Model file for the job. Use its own axes, mm. A direction names the side the tool comes from. Coordinates: 2 decimals unless noted, no trailing zeros. Write each loop counter-clockwise with the first axis right and the second up, starting at its lowest first coordinate (ties: lowest second). Pieces come first, ordered by that corner, then holes. Notation, with made-up numbers: (11, -15) - (25, -15) arc R19 cw to (25, -4) - close; hole circle Ø6 at (-6, 32). An arc over 180 degrees is marked (long way). Put each result on its own line as item: value. Start each with the question number.
1. Drop flat-ended pins along their axis: P1, Ø12, axis at x = 31, y = 47.5, coming from the +Z side; P2, Ø4, axis at x = 29.5, z = 14.5, coming from the +Y side; P3, Ø4.5, axis at x = 17.5, z = 23, coming from the -Y side; P4, Ø13, axis at y = 24.5, z = 20, coming from the -X side. Give the stop position or say it passes through.
2. Pull direction Z, two halves, no side cores. Call faces 1 (the face through (15.029, 2.535, 21.425)), 2 (the face through (50, 53, 21)), 3 (the face through (56, 38, 37)), 4 (the face through (60, 27, 18)): released by +Z, released by -Z, zero draft, split by the parting line, or undercut.
3. Saw through at A-A, the plane x = 47.5. Write the cut outline in (y, z), plus the area to 3 significant figures.
4. Saw through at B-B, the plane y = 45.5. Write the cut outline in (x, z), plus the area to 4 significant figures.
5. Drill centre lines: L1, parallel to X at y = 14, z = 30; L2, parallel to X at y = 1, z = 23; L3, parallel to X at y = 13, z = 31. Where is each one in solid material? Low to high. Write a range as from..to.
6. Saw through at C-C, the plane z = 27. Write the cut outline in (x, y), plus the area to 3 significant figures.
7. Which spindle directions (+Z, -Z, +X, -X, +Y, -Y) get a long thin tool onto all of the face, cutting with end or side? Do faces 5 (the face through (50, 50, 29)), 6 (the face through (10, 28, 17)), 7 (the face through (24, 40, 14)). Say none if no direction does.
8. Saw through at D-D, the plane y = 33. Write the cut outline in (x, z).
Autodesk Inventor part; units mm, degrees
ref_plane "YZ Plane" through (0, 0, 0) normal (1, 0, 0) x (0, 1, 0)
ref_plane "XZ Plane" through (0, 0, 0) normal (0, 1, 0) x (-1, 0, 0)
ref_plane "XY Plane" through (0, 0, 0) normal (0, 0, 1) x (1, 0, 0)
sketch "Sketch3" plane through (0, 0, 0) normal (0, 0, 1) x (1, 0, 0)
  line L0 (0, 0) -> (0, 55)
  line L1 (0, 55) -> (17.5, 55)
  line L2 (17.5, 55) -> (17.5, 40)
  line L3 (17.5, 40) -> (45, 40)
  line L4 (45, 40) -> (45, 55)
  line L5 (10.4377, 0) -> (0, 0)
  line L6 (45, 55) -> (60, 55)
  line L7 (60, 55) -> (60, 0)
  line L8 (60, 0) -> (0, 0)
  dimension "d7" = 55
  dimension "d8" = 17.5
  dimension "d12" = 15
  dimension "d13" = 27.5
  dimension "d14" = 15
  dimension "d15" = 55
  dimension "d16" = 60
extrude "Extrusion2" add sketch "Sketch3" along normal blind 5
sketch "Sketch4" plane through (0, 55, 0) normal (0, 1, 0) x (1, 0, 0)
  line L0 (17.5, -5) -> (0, -5)
  line L1 (0, -37) -> (17.5, -37)
  line L2 (17.5, -37) -> (17.5, -5)
  line L3 (17.5, -5) -> (0, -5)
  line L4 (0, -5) -> (0, -37)
  point P0 (0, 0)
  dimension "d20" = 32
  dimension "d21" = 17.5
extrude "Extrusion3" add sketch "Sketch4" against normal blind 55
sketch "Sketch5" plane through (45, 55, 0) normal (0, 1, 0) x (1, 0, 0)
  line L0 (15, 0) -> (15, -5)
  line L1 (-0.039, -37) -> (15, -37)
  line L2 (15, -37) -> (15, -5)
  line L3 (15, -5) -> (-0.039, -5)
  line L4 (-0.039, -5) -> (-0.039, -37)
  point P0 (-45, 0)
  dimension "d24" = 32
extrude "Extrusion4" add sketch "Sketch5" against normal blind 5
sketch "Sketch7" plane through (17.5, 40, 0) normal (0, 1, 0) x (1, 0, 0)
  line L0 (0, -5) -> (0, -37)
  line L1 (27.5, -5) -> (0, -5)
  line L2 (0, -37) -> (7.5, -37)
  line L3 (7.5, -37) -> (7.5, -5)
  line L4 (7.5, -5) -> (0, -5)
  line L5 (0, -5) -> (0, -37)
  point P0 (-17.5, 0)
  dimension "d27" = 7.5
extrude "Extrusion5" add sketch "Sketch7" against normal blind 40
sketch "Sketch8" plane through (0, 0, 5) normal (0, 0, 1) x (1, 0, 0)
  line L0 (25, 0) -> (60, 0)
  line L1 (60, 0) -> (60, 50)
  line L2 (25, 0) -> (60, 0)
  line L3 (60, 0) -> (60, 5)
  line L4 (60, 5) -> (25, 5)
  line L5 (25, 5) -> (25, 0)
  point P0 (0, 0)
  dimension "d30" = 5
extrude "Extrusion6" add sketch "Sketch8" along normal blind 32
sketch "Sketch9" plane through (0, 0, 5) normal (0, 0, 1) x (1, 0, 0)
  line L0 (60, 50) -> (45, 50)
  line L1 (60, 50) -> (55, 50)
  line L2 (55, 50) -> (55, 0)
  line L3 (55, 0) -> (60, 0)
  line L4 (60, 0) -> (60, 50)
  point P0 (0, 0)
  dimension "d31" = 32
  dimension "d33" = 50
  dimension "d34" = 5
extrude "Extrusion7" add sketch "Sketch9" along normal blind 32
sketch "Sketch10" plane through (0, 55, 0) normal (0, 1, 0) x (1, 0, 0)
  line L0 (10, -30.5) -> (5, -30.5)
  line L1 (5, -30.5) -> (5, -4.5)
  line L2 (5, -4.5) -> (10, -4.5)
  line L3 (10, -4.5) -> (10, -30.5)
  line L4 (17.5, 0) -> (17.5, -37)
  line L5 (0, 0) -> (17.5, 0)
  line L6 (0, 0) -> (0, -37)
  dimension "d45" = 5
  dimension "d46" = 26
  dimension "d47" = 7.5
  dimension "d48" = 4.5
extrude "Extrusion8" cut sketch "Sketch10" against normal blind 60
sketch "Sketch11" plane through (0, 55, 0) normal (0, 1, 0) x (1, 0, 0)
  line L0 (5, -4.5) -> (5, -30.5)
  line L1 (0, 0) -> (0, -37)
  line L2 (5, -28) -> (0, -28)
  line L3 (0, -28) -> (0, -7)
  line L4 (0, -7) -> (5, -7)
  line L5 (5, -7) -> (5, -28)
  line L6 (0, -37) -> (17.5, -37)
  point P0 (5, -35)
  dimension "d52" = 21
  dimension "d53" = 9
extrude "Extrusion9" cut sketch "Sketch11" against normal blind 60
sketch "Sketch12" plane through (0, 0, 0) normal (0, -1, 0) x (1, 0, 0)
  circle A0 centre (17.5, 10.5) radius 2.5
  circle A1 centre (17.5, 23) radius 2.5
  line L0 (10, 30.5) -> (10, 4.5)
  line L1 (0, 37) -> (60, 37)
  line L2 (60, 0) -> (0, 0)
  point P0 (10, 35)
  point P1 (25, 35)
  dimension "d56" = 5
  dimension "d57" = 5
  dimension "d58" = 7.5
  dimension "d59" = 7.5
  dimension "d78" = 14
  dimension "d79" = 12.5
hole "Hole1" at (17.5, 0, 10.5) at (17.5, 0, 23) direction (0, 1, 0) diameter 5.86 depth 5 tip angle 118
sketch "Sketch14" plane through (0, 55, 37) normal (0, 0, 1) x (1, 0, 0)
  line L0 (55, -5) -> (55, -50)
  line L1 (60, 0) -> (60, -55)
  line L2 (55, -50) -> (60, -50)
  line L3 (60, -50) -> (60, -45)
  line L4 (60, -45) -> (55, -45)
  line L5 (55, -45) -> (55, -50)
  point P0 (0, -55)
  dimension "d69" = 5
extrude "Extrusion10" cut sketch "Sketch14" along normal mid plane 64
sketch "Sketch20" plane through (45, 55, 0) normal (0, 1, 0) x (1, 0, 0)
  line L0 (-0.039, -37) -> (-0.039, -5)
  line L1 (0, 0) -> (15, 0)
  line L2 (-0.039, -21) -> (10, -21)
  line L3 (10, -21) -> (10, 0)
  line L4 (10, 0) -> (-0.039, 0)
  line L5 (-0.039, 0) -> (-0.039, -21)
  line L6 (15, 0) -> (15, -37)
  point P0 (-45, 0)
  dimension "d77" = 5
extrude "Extrusion12" cut sketch "Sketch20" against normal blind 15
properties part number "Holder" material "Iron, Cast"
Final values:
1. P1: passes through
1. P2: stops at y = 5
1. P3: stops at y = 5.41
1. P4: stops at x = 10
2. face 1: undercut
2. face 2: released by -Z
2. face 3: released by +Z
2. face 4: zero draft
3. outline: (0, 0) - (40, 0) - (40, 5) - (5, 5) - (5, 37) - (0, 37) - close; (50, 21) - (55, 21) - (55, 37) - (50, 37) - close
3. area: 440 mm²
4. outline: (0, 0) - (17.5, 0) - (17.5, 37) - (0, 37) - (0, 28) - (5, 28) - (5, 30.5) - (10, 30.5) - (10, 4.5) - (5, 4.5) - (5, 7) - (0, 7) - close; (55, 0) - (60, 0) - (60, 37) - (55, 37) - close
4. area: 597.5 mm²
5. L1: x = 0..5, 10..25, 55..60
5. L2: x = 10..14.57, 20.43..60
5. L3: x = 0..25, 55..60
6. outline: (10, 0) - (60, 0) - (60, 5) - (25, 5) - (25, 40) - (17.5, 40) - (17.5, 55) - (10, 55) - close; (44.96, 50) - (55, 50) - (55, 10) - (60, 10) - (60, 55) - (44.96, 55) - close
6. area: 1,160 mm²
7. face 5: +Z, -Z
7. face 6: +Y, -Y
7. face 7: +Z, -Z, +Y
8. outline: (0, 0) - (60, 0) - (60, 37) - (55, 37) - (55, 5) - (25, 5) - (25, 37) - (0, 37) - (0, 28) - (5, 28) - (5, 30.5) - (10, 30.5) - (10, 4.5) - (5, 4.5) - (5, 7) - (0, 7) - close
